For this review, take the finished solid that the model builds, in its own axes (mm). Round coordinates to 2 decimals unless told otherwise and drop trailing zeros. Write each loop counter-clockwise with the first axis right and the second up, starting at its lowest first coordinate (ties: lowest second). Pieces come first, ordered by that corner, then holes. Notation, with made-up numbers: M 30.25,11.25 L 39.25,11.25 A29 ccw 39.25,32.25 Z; hole C 83,-13 d10. An arc over 180 degrees is marked long. Answer in a Markdown table with one row per item.
Autodesk Inventor part; units mm, degrees
ref_plane "YZ Plane" through (0, 0, 0) normal (1, 0, 0) x (0, 1, 0)
ref_plane "XZ Plane" through (0, 0, 0) normal (0, 1, 0) x (-1, 0, 0)
ref_plane "XY Plane" through (0, 0, 0) normal (0, 0, 1) x (1, 0, 0)
sketch "Sketch1" plane through (0, 0, 0) normal (0, 0, 1) x (1, 0, 0)
  line L0 (1033.8246, 340.1521) -> (1033.8246, -117.0479)
  line L1 (627.4246, -117.0479) -> (627.4246, 340.1521)
  line L2 (627.4246, -117.0479) -> (1033.8246, -117.0479)
  arc A0 (665.5246, 340.1521) -> (995.7246, 340.1521) centre (830.6246, 678.8187) ccw
  line L3 (627.4246, 340.1521) -> (665.5246, 340.1521)
  line L4 (995.7246, 340.1521) -> (1033.8246, 340.1521)
  point P0 (0, 0)
  dimension "d0" = 406.4
  dimension "d1" = 457.2
extrude "Extrusion1" add sketch "Sketch1" along normal blind 19.05
sketch "Sketch2" plane through (0, 0, 19.05) normal (0, 0, 1) x (1, 0, 0)
  line L0 (1033.8246, 340.1521) -> (627.4246, 340.1521)
  line L1 (627.4246, -117.0479) -> (-960.0754, -117.0479)
  line L2 (627.4246, 340.1521) -> (646.4746, 340.1521)
  line L3 (646.4746, 340.1521) -> (646.4746, -117.0479)
  line L4 (646.4746, -117.0479) -> (627.4246, -117.0479)
  line L5 (627.4246, -117.0479) -> (627.4246, 340.1521)
  line L6 (1033.8246, -117.0479) -> (1033.8246, 340.1521)
  line L7 (1033.8246, 340.1521) -> (1014.7746, 340.1521)
  line L8 (1014.7746, 340.1521) -> (1014.7746, -117.0479)
  line L9 (1014.7746, -117.0479) -> (1033.8246, -117.0479)
  line L10 (1033.8246, -117.0479) -> (1033.8246, 340.1521)
  line L11 (627.4246, 340.1521) -> (627.4246, -117.0479)
  line L12 (627.4246, 263.9521) -> (646.4746, 263.9521)
  line L13 (1014.7746, 263.9521) -> (1033.8246, 263.9521)
  line L14 (627.4246, 187.7521) -> (646.4746, 187.7521)
  line L15 (1014.7746, 187.7521) -> (1033.8246, 187.7521)
  line L16 (627.4246, 111.5521) -> (646.4746, 111.5521)
  line L17 (1014.7746, 111.5521) -> (1033.8246, 111.5521)
  line L18 (627.4246, 35.3521) -> (646.4746, 35.3521)
  line L19 (1014.7746, 35.3521) -> (1033.8246, 35.3521)
  line L20 (1033.8246, -40.8479) -> (1014.7746, -40.8479)
  line L21 (646.4746, -40.8479) -> (627.4246, -40.8479)
  point P0 (0, 0)
  dimension "d7" = 19.05
  dimension "d8" = 19.05
extrude "Extrusion2" cut sketch "Sketch2" against normal blind 19.05 contours L6 L13 L8 L0 | L3 L12 L5 L0 | L6 L17 L8 L15 | L3 L16 L5 L14 | L6 L20 L8 L19 | L3 L21 L5 L18
sketch "Sketch3" plane through (0, 0, 19.05) normal (0, 0, 1) x (1, 0, 0)
  line L0 (1131.5205, 302.0521) -> (511.2286, 302.0521)
  line L1 (1014.7746, 340.1521) -> (995.7246, 340.1521)
  line L2 (1127.4261, 283.0021) -> (305.147, 283.0021)
  line L3 (830.6246, 74.0239) -> (830.6246, 388.6053)
  line L4 (1033.8246, 187.7521) -> (1033.8246, 263.9521)
  line L5 (983.0246, 283.0021) -> (881.4246, 283.0021)
  line L6 (881.4246, 283.0021) -> (881.4246, 263.9521)
  line L7 (881.4246, 263.9521) -> (983.0246, 263.9521)
  line L8 (983.0246, 263.9521) -> (983.0246, 283.0021)
  line L9 (1014.7746, 263.9521) -> (1014.7746, 340.1521)
  line L10 (678.2246, 283.0021) -> (779.8246, 283.0021)
  line L11 (779.8246, 283.0021) -> (779.8246, 263.9521)
  line L12 (779.8246, 263.9521) -> (678.2246, 263.9521)
  line L13 (678.2246, 263.9521) -> (678.2246, 283.0021)
  line L14 (646.4746, 340.1521) -> (646.4746, 263.9521)
  point P0 (0, 0)
  dimension "d24" = 38.1
  dimension "d25" = 19.05
  dimension "d26" = 203.2
  dimension "d27" = 31.75
  dimension "d28" = 101.6
  dimension "d29" = 19.05
  dimension "d30" = 31.75
  dimension "d31" = 101.6
  dimension "d32" = 19.05
extrude "Extrusion3" cut sketch "Sketch3" against normal blind 25.4 contours L8 L7 L6 L2 | L11 L12 L13 L2
properties part number "right side" material "Wood (Birch)"
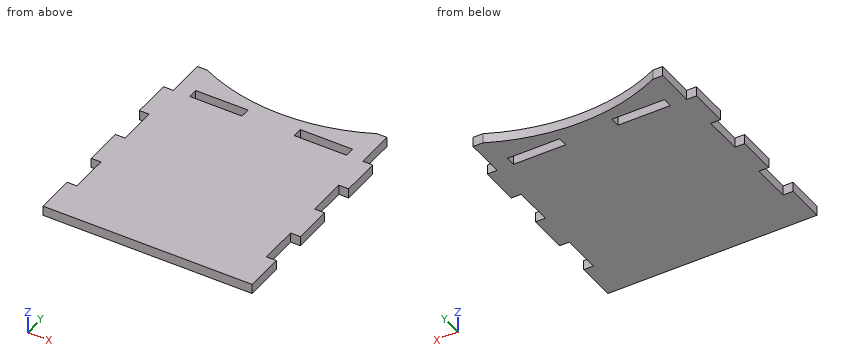
Q1. Take a section at C-C (y = 17). State the section outline as (x, z) points.
Found:
| item | result |
|---|---|
| outline | M 646.47,0 L 1014.77,0 L 1014.77,19.05 L 646.47,19.05 Z |
Q2. Take a section at B-B (z = 6.5). State how many separate pieces and enclosed holes the cut face has, then the cut area to 3 significant figures.
Found:
| item | result |
|---|---|
| separate pieces | 1 |
| enclosed holes | 2 |
| area | 165,000 mm² |
Q3. Insertion check: P1, Ø9.5, axis at x = 1021.5, z = 13.5, coming from the +Y side; P2, Ø5.5, axis at y = -14, z = 10, coming from the +X side; P3, Ø5, axis at y = 120, z = 8, coming from the -X side. Each pin has a flat end and moves straight along its axis. Give the tip position at first contact, or say it passes through.
Found:
| item | result |
|---|---|
| P1 | y = 263.95 |
| P2 | x = 1014.77 |
| P3 | x = 646.47 |
Q4. Take a section at D-D (x = 854). State the section outline as (y, z) points, then the cut area to 3 significant figures.
Found:
| item | result |
|---|---|
| outline | M -117.05,0 L 302.78,0 L 302.78,19.05 L -117.05,19.05 Z |
| area | 8,000 mm² |
Q5. For probe 1 along X at (y, z) = (278.5, 17); probe 2 along Y at (x, z) = (831, 1.25); probe 3 along X at (y, z) = (28, 6.5), list the stretches that pass through material, from the lowest coordinate up.
Found:
| item | result |
|---|---|
| probe 1 | 646.47 to 678.22, 779.82 to 881.42, 983.02 to 1014.77 |
| probe 2 | -117.05 to 302.05 |
| probe 3 | 646.47 to 1014.77 |
Q6. Take a section at A-A (x = 918). State the section outline as (y, z) points.
Found:
| item | result |
|---|---|
| outline | M -117.05,0 L 263.95,0 L 263.95,19.05 L -117.05,19.05 Z; M 283,0 L 312.32,0 L 312.32,19.05 L 283,19.05 Z |
